Here's how the part is built. I have some questions about the finished solid (model axes, mm). Give positions to 0.01 mm unless a question says otherwise; leave off trailing zeros. Write each loop counter-clockwise with the first axis right and the second up, starting at its lowest first coordinate (ties: lowest second). Pieces come first, ordered by that corner, then holes. Notation, with made-up numbers: (-10, 20) -> (28, 20) arc R9 ccw to (28, 33) -> close; hole circle Ø3 at (-3, -28). An arc over 180 degrees is marked (long way). Return JSON: item names as keys, results as strings.
from build123d import *

# Parameters (mm, degrees)
F0_W     = 355.6
F0_H     = 228.6
F1_DEPTH = 12.7
F2_W     = 12.7
F2_H     = 12.7
F3_DEPTH = 25.4
F4_W     = 330.2
F4_H     = 6.35
F5_DEPTH = 6.35


with BuildPart() as f1:
    # F0 (on Front) → F1 (new body)
    with BuildSketch(Plane.XZ):
        with Locations((177.8, 114.3)):
            Rectangle(F0_W, F0_H)
    extrude(amount=F1_DEPTH)

    # F2 (on face) → F3 (cut)
    with BuildSketch(Plane.XZ.offset(12.7)):
        with Locations((6.35, 222.25)):
            Rectangle(F2_W, F2_H)
        with Locations((6.35, 196.85)):
            Rectangle(F2_W, F2_H)
        with Locations((6.35, 171.45)):
            Rectangle(F2_W, F2_H)
        with Locations((6.35, 146.05)):
            Rectangle(F2_W, F2_H)
        with Locations((6.35, 120.65)):
            Rectangle(F2_W, F2_H)
        with Locations((6.35, 95.25)):
            Rectangle(F2_W, F2_H)
        with Locations((6.35, 69.85)):
            Rectangle(F2_W, F2_H)
        with Locations((6.35, 44.45)):
            Rectangle(F2_W, F2_H)
        with Locations((6.35, 19.05)):
            Rectangle(F2_W, F2_H)
        Polygon((346.075, 228.6), (342.9, 228.6), (342.9, 215.9), (346.075, 215.9), (352.425, 215.9), (355.6, 215.9), (355.6, 228.6), (352.425, 228.6), align=None)
        with Locations((349.25, 196.786214)):
            Rectangle(F2_W, F2_H)
        with Locations((349.25, 171.386214)):
            Rectangle(F2_W, F2_H)
        with Locations((349.25, 145.986214)):
            Rectangle(F2_W, F2_H)
        with Locations((349.25, 120.586214)):
            Rectangle(F2_W, F2_H)
        with Locations((349.25, 95.186214)):
            Rectangle(F2_W, F2_H)
        with Locations((349.25, 69.786214)):
            Rectangle(F2_W, F2_H)
        with Locations((349.25, 44.386214)):
            Rectangle(F2_W, F2_H)
        with Locations((349.25, 18.986214)):
            Rectangle(F2_W, F2_H)
    extrude(amount=-F3_DEPTH, mode=Mode.SUBTRACT)

    # F4 (on face) → F5 (cut)
    with BuildSketch(Plane(origin=(0, 0, 0), x_dir=(-1, 0, 0), z_dir=(0, 1, 0))):
        with Locations((-177.8, 15.875)):
            Rectangle(F4_W, F4_H)
    extrude(amount=-F5_DEPTH, mode=Mode.SUBTRACT)


solid = f1.part
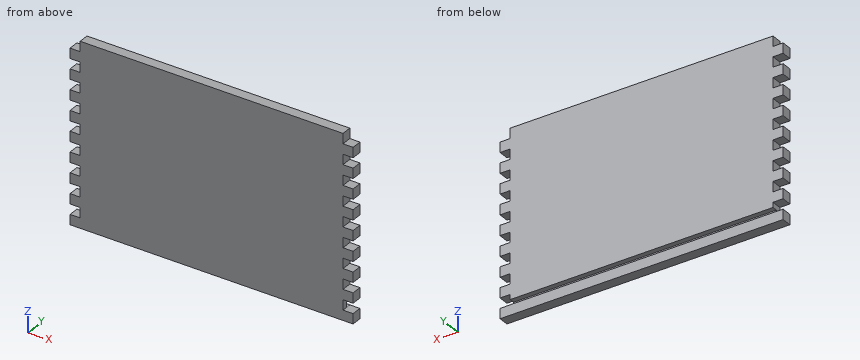
1. Suppose I cut it at A-A, the plane z = 70.5. List the corners of the cut face in (x, y) for me.
Taken from the geometry:
{"outline": "(12.7, -12.7) -> (342.9, -12.7) -> (342.9, 0) -> (12.7, 0) -> close"}
2. If I drill on line 1 (Z direction, x = 198, y = -5.5); line 2 (X direction, y = -11.25, z = 119), over which ranges is the centre line in solid material (lowest first)? Write a range as [from, to].
Taken from the geometry:
{"line 1": "z = [0, 12.7], [19.05, 228.6]", "line 2": "x = [12.7, 342.9]"}
3. For pin 1 Ø6.5 at (y, z) = (-5.5, 224) entering from +X; pin 2 Ø3 at (x, z) = (164.5, 141) entering from +Y; pin 3 Ø4 at (y, z) = (-6.5, 19.5) entering from -X; pin 4 Ø6.5 at (x, y) = (5.5, -5.5) entering from +Z, each with a flat end and sliding along its axis, tell me the tip position at first contact or that it passes through.
Taken from the geometry:
{"pin 1": "stops at x = 342.9", "pin 2": "stops at y = 0", "pin 3": "stops at x = 12.7", "pin 4": "stops at z = 215.9"}
